```python
from build123d import *
from OCP.BRepFilletAPI import BRepFilletAPI_MakeChamfer

# Parameters (mm, degrees)
SKETCH1_W                 = 41.91
SKETCH1_H                 = 41.91
EXTRUDE1_DEPTH            = 33
SKETCH9_R                 = 11
EXTRUDE5_DEPTH            = 2
SKETCH7_R                 = 2.50063
EXTRUDE3_DEPTH            = 18
F_4_40_TAPPED_HOLE1_D     = 2.2606
F_4_40_TAPPED_HOLE1_DEPTH = 6.41
F_4_40_TAPPED_HOLE1_TIP   = 0.679152758
F_4_40_TAPPED_HOLE2_D     = 2.2606
F_4_40_TAPPED_HOLE2_DEPTH = 29.905
F_4_40_TAPPED_HOLE2_TIP   = 0.679152758
SKETCH14_R                = 3.1
CUT_EXTRUDE1_DEPTH        = 2.6
CHAMFER1_SIZE             = 0.508
CHAMFER2_SIZE             = 4.064
SKETCH16_R                = 3.3147
CUT_EXTRUDE3_DEPTH        = 5.08
BOSS_EXTRUDE1_START       = 4.08
SKETCH17_R                = 2.50063
BOSS_EXTRUDE1_DEPTH       = 4.08
CHAMFER3_SIZE             = 0.254
CHAMFER4_SIZE             = 0.254
CHAMFER4_SIZE2            = 0.205559306
SKETCH18_W                = 5.00126
SKETCH18_H                = 1
CUT_EXTRUDE4_DEPTH        = 15
SKETCH24_R                = 0.5
BOSS_EXTRUDE2_DEPTH       = 19
SKETCH25_R                = 5.83
BOSS_EXTRUDE3_DEPTH       = 14
SKETCH26_R                = 17.29
BOSS_EXTRUDE4_DEPTH       = 11
SKETCH27_R                = 17.29
SKETCH27_R_2              = 5.83
CUT_EXTRUDE5_DEPTH        = 6


with BuildPart() as part:
    # Sketch1 → Extrude1 (new body)
    with BuildSketch(Plane(origin=(0, 0, 0), x_dir=(1, 0, 0), z_dir=(0, 1, 0))):
        Rectangle(SKETCH1_W, SKETCH1_H)
    extrude(amount=-EXTRUDE1_DEPTH)

    # Sketch9 → Extrude5 (add)
    with BuildSketch(Plane(origin=(0, 0, 0), x_dir=(1, 0, 0), z_dir=(0, 1, 0))):
        with Locations(Location((0, 0, 0), (0, 0, 90))):
            Circle(SKETCH9_R)
    extrude(amount=EXTRUDE5_DEPTH)

    # Sketch7 → Extrude3 (add)
    with BuildSketch(Plane(origin=(0, 2, 0), x_dir=(-1, 0, 0), z_dir=(0, 1, 0))):
        with Locations(Location((0, 0, 0), (0, 0, 90))):
            Circle(SKETCH7_R)
    extrude(amount=EXTRUDE3_DEPTH)

    # #4-40 Tapped Hole1
    with Locations(Plane(origin=(0, 0, 0), x_dir=(-1, 0, 0), z_dir=(0, 1, 0))):
        with Locations((15.5, -15.5), (15.5, 15.5), (-15.5, 15.5), (-15.5, -15.5)):
            Hole(F_4_40_TAPPED_HOLE1_D / 2, depth=F_4_40_TAPPED_HOLE1_DEPTH)
            with Locations((0, 0, -(F_4_40_TAPPED_HOLE1_DEPTH + F_4_40_TAPPED_HOLE1_TIP / 2))):  # 118° drill point
                Cone(0, F_4_40_TAPPED_HOLE1_D / 2, F_4_40_TAPPED_HOLE1_TIP, mode=Mode.SUBTRACT)

    # #4-40 Tapped Hole2
    with Locations(Plane.XZ.offset(33)):
        with Locations((15.5, -15.5), (-15.5, 15.5), (-15.5, -15.5), (15.5, 15.5)):
            Hole(F_4_40_TAPPED_HOLE2_D / 2, depth=F_4_40_TAPPED_HOLE2_DEPTH)
            with Locations((0, 0, -(F_4_40_TAPPED_HOLE2_DEPTH + F_4_40_TAPPED_HOLE2_TIP / 2))):  # 118° drill point
                Cone(0, F_4_40_TAPPED_HOLE2_D / 2, F_4_40_TAPPED_HOLE2_TIP, mode=Mode.SUBTRACT)

    # Sketch14 → Cut-Extrude1 (cut)
    with BuildSketch(Plane(origin=(0, -33, 0), x_dir=(1, 0, 0), z_dir=(0, 1, 0))):
        with Locations(Location((15.5, 15.5, 0), (0, 0, 270))):
            Circle(SKETCH14_R)
        with Locations(Location((-15.5, 15.5, 0), (0, 0, 270))):
            Circle(SKETCH14_R)
        with Locations(Location((-15.5, -15.5, 0), (0, 0, 270))):
            Circle(SKETCH14_R)
        with Locations(Location((15.5, -15.5, 0), (0, 0, 270))):
            Circle(SKETCH14_R)
    extrude(amount=CUT_EXTRUDE1_DEPTH, mode=Mode.SUBTRACT)

    # Chamfer1
    chamfer1_edges = [part.edges().sort_by_distance(p)[0] for p in [
        (0, 20, -2.50063),
    ]]
    chamfer(chamfer1_edges, length=CHAMFER1_SIZE)

    # Chamfer2
    chamfer2_edges = [part.edges().sort_by_distance(p)[0] for p in [
        (20.955, -16.5, 20.955),
        (-20.955, -16.5, 20.955),
        (-20.955, -16.5, -20.955),
        (20.955, -16.5, -20.955),
    ]]
    chamfer(chamfer2_edges, length=CHAMFER2_SIZE)

    # Sketch16 → Cut-Extrude3 (cut)
    with BuildSketch(Plane.XZ.offset(33)):
        with Locations(Location((0, 0, 0), (0, 0, 270))):
            Circle(SKETCH16_R)
    extrude(amount=-CUT_EXTRUDE3_DEPTH, mode=Mode.SUBTRACT)

    # Sketch17 → Boss-Extrude1 (add)
    with BuildSketch(Plane.XZ.offset(27.92).offset(BOSS_EXTRUDE1_START)):
        with Locations(Location((0, 0, 0), (0, 0, 90))):
            Circle(SKETCH17_R)
    extrude(amount=-BOSS_EXTRUDE1_DEPTH)

    # Chamfer3
    chamfer3_edges = [part.edges().sort_by_distance(p)[0] for p in [
        (-18.923, -33, 18.923),
        (0, -33, 3.3147),
        (0, -32, -2.50063),
        (-20.955, 0, 0),
        (-20.955, -33, 0),
        (20.955, 0, 0),
        (0, 0, -20.955),
        (0, 0, 20.955),
        (-18.923, 0, -18.923),
        (18.923, 0, -18.923),
        (18.923, 0, 18.923),
        (-18.923, 0, 18.923),
        (0, -33, 20.955),
        (20.955, -33, 0),
        (0, -33, -20.955),
        (-18.923, -33, -18.923),
        (18.923, -33, -18.923),
        (18.923, -33, 18.923),
    ]]
    chamfer(chamfer3_edges, length=CHAMFER3_SIZE)

    # Chamfer4: one chamfer whose edges measure the first distance from different faces: ONE call of the kernel's chamfer builder (chamfer() names one face for all edges)
    chamfer4_edges_1 = [part.edges().sort_by_distance(p)[0] for p in [
        (16.891, -16.5, -20.955),
        (20.955, -16.5, -16.891),
    ]]
    chamfer4_side_1 = [part.faces().sort_by_distance(p)[0] for p in [
        (18.923, -16.5, -18.923),
    ]]
    chamfer4_edges_2 = [part.edges().sort_by_distance(p)[0] for p in [
        (-16.891, -16.5, -20.955),
        (-20.955, -16.5, -16.891),
    ]]
    chamfer4_side_2 = [part.faces().sort_by_distance(p)[0] for p in [
        (-18.923, -16.5, -18.923),
    ]]
    chamfer4_edges_3 = [part.edges().sort_by_distance(p)[0] for p in [
        (20.955, -16.5, 16.891),
        (16.891, -16.5, 20.955),
    ]]
    chamfer4_side_3 = [part.faces().sort_by_distance(p)[0] for p in [
        (18.923, -16.5, 18.923),
    ]]
    chamfer4_edges_4 = [part.edges().sort_by_distance(p)[0] for p in [
        (-16.891, -16.5, 20.955),
        (-20.955, -16.5, 16.891),
    ]]
    chamfer4_side_4 = [part.faces().sort_by_distance(p)[0] for p in [
        (-18.923, -16.5, 18.923),
    ]]
    chamfer4 = BRepFilletAPI_MakeChamfer(part.part.solid().wrapped)
    for e in chamfer4_edges_1:
        chamfer4.Add(CHAMFER4_SIZE, CHAMFER4_SIZE2, e.wrapped, chamfer4_side_1[0].wrapped)  # the first distance lies on this face
    for e in chamfer4_edges_2:
        chamfer4.Add(CHAMFER4_SIZE, CHAMFER4_SIZE2, e.wrapped, chamfer4_side_2[0].wrapped)  # the first distance lies on this face
    for e in chamfer4_edges_3:
        chamfer4.Add(CHAMFER4_SIZE, CHAMFER4_SIZE2, e.wrapped, chamfer4_side_3[0].wrapped)  # the first distance lies on this face
    for e in chamfer4_edges_4:
        chamfer4.Add(CHAMFER4_SIZE, CHAMFER4_SIZE2, e.wrapped, chamfer4_side_4[0].wrapped)  # the first distance lies on this face
    add(Compound.cast(chamfer4.Shape()), mode=Mode.REPLACE)

    # Sketch18 → Cut-Extrude4 (cut)
    with BuildSketch(Plane(origin=(0, 20, 0), x_dir=(1, 0, 0), z_dir=(0, 1, 0))):
        with Locations((0, 2.50063)):
            Rectangle(SKETCH18_W, SKETCH18_H)
    extrude(amount=-CUT_EXTRUDE4_DEPTH, mode=Mode.SUBTRACT)

    # Sketch24 → Boss-Extrude2 (add)
    with BuildSketch(Plane(origin=(20.955, 0, 0), x_dir=(0, 0, -1), z_dir=(1, 0, 0))):
        with Locations((2.4, -30.086520784)):
            Circle(SKETCH24_R)
        with Locations((1.2, -30.086520784)):
            Circle(SKETCH24_R)
        with Locations((0, -30.086520784)):
            Circle(SKETCH24_R)
    extrude(amount=BOSS_EXTRUDE2_DEPTH)

    # Sketch25 → Boss-Extrude3 (add)
    with BuildSketch(Plane(origin=(0, 20, 0), x_dir=(1, 0, 0), z_dir=(0, 1, 0))):
        with Locations(Location((0, 0, 0), (0, 0, 270))):
            Circle(SKETCH25_R)
    extrude(amount=-BOSS_EXTRUDE3_DEPTH)

    # Sketch26 → Boss-Extrude4 (add)
    with BuildSketch(Plane(origin=(0, 20, 0), x_dir=(1, 0, 0), z_dir=(0, 1, 0))):
        with Locations(Location((0, 0, 0), (0, 0, 270))):
            Circle(SKETCH26_R)
    extrude(amount=-BOSS_EXTRUDE4_DEPTH)

    # Sketch27 → Cut-Extrude5 (cut)
    with BuildSketch(Plane(origin=(0, 20, 0), x_dir=(1, 0, 0), z_dir=(0, 1, 0))):
        with Locations(Location((0, 0, 0), (0, 0, 270))):
            Circle(SKETCH27_R)
        with Locations(Location((0, 0, 0), (0, 0, 270))):
            Circle(SKETCH27_R_2, mode=Mode.SUBTRACT)
    extrude(amount=-CUT_EXTRUDE5_DEPTH, mode=Mode.SUBTRACT)


solid = part.part
```
The listing builds one solid part. Answer for the finished solid, in the listing's coordinates (mm). A direction names the side the tool comes from. Round coordinates to 2 decimals unless told otherwise and drop trailing zeros. Loops run counter-clockwise (first coordinate to the right, second up) from the corner with the lowest first, then second, coordinate; pieces in that order, holes last. Notation, with made-up numbers: (12.25, 68) - (33.25, 68) arc R26 ccw to (33.25, 95) - close; hole circle Ø11 at (78, 55). An arc over 180 degrees is marked (long way). Return JSON: item names as keys, results as strings. Group by question number.
1. The part is cut by section D-D on x = 27.5. Determine the outline of the cut face in (y, z).
2. Each of these flat-tipped pins is pushed along its axis until it touches: P1, Ø3.5, axis at x = -15.5, z = 15.5, coming from the +Y side; P2, Ø1.9, axis at x = 16.5, z = 16.5, coming from the -Y side; P3, Ø1.8, axis at x = -15.5, z = -15.5, coming from the -Y side; P4, Ø4, axis at x = 0, z = 0, coming from the -Y side. Where does it stop, or does it pass through?
3. Consider probe 1 along X at (y, z) = (-2, 15.5) (3 decimals); probe 2 along X at (y, z) = (-5, -15) (3 decimals). Determine where each line is inside the solid, lowest interval first.
4. The part is cut by section B-B on x = -15.5. Determine the outline of the cut face in (y, z) (3 decimals), then the cut area to 3 significant figures.
5. The mould has two halves that part along Z. Classify faces 1 (the cylindrical face through (-0.751, -29.86, 2.385)), 2 (the flat face through (-18.86, -0.13, 18.81)), 3 (the flat face through (0, 20, 0)): pulls with the +Z half, pulls with the -Z half, needs draft (parallel to the pull), parting line crosses it, or undercut.
6. The part is cut by section A-A on x = 10. Determine the outline of the cut face in (y, z) (3 decimals), then the cut area to 3 significant figures.
7. Which of the six approach directions +Z, -Z, +X, -X, +Y, -Y give full straight-line access (tool end or side, diameter ignored) to faces 4 (the flat face through (-18.897, -16.273, 18.949)), 5 (the cylindrical face through (10.74, 0.99, 2.38)), 6 (the flat face through (0, -32, 0))?
8. The part is cut by section C-C on y = 10.5. Determine the outline of the cut face in (x, z).
Resolved:
{
 "1": {"outline": "circle Ø1 at (-30.09, -2.4); circle Ø1 at (-30.09, -1.2); circle Ø1 at (-30.09, 0)"},
 "2": {"P1": "stops at y = 0", "P2": "stops at y = -30.4", "P3": "passes through", "P4": "stops at y = -32"},
 "3": {"probe 1": "x = -20.955 to -16.63, -14.37 to 14.37, 16.63 to 20.955", "probe 2": "x = -20.955 to -16.514, -14.486 to 14.486, 16.514 to 20.955"},
 "4": {"outline": "(-33, -20.701) - (-32.746, -20.955) - (-0.254, -20.955) - (0, -20.701) - (0, -16.63) - (-30.4, -16.63) - (-30.4, -18.6) - (-33, -18.6) - close; (-33, -12.4) - (-30.4, -12.4) - (-30.4, -14.37) - (0, -14.37) - (0, 14.37) - (-30.4, 14.37) - (-30.4, 12.4) - (-33, 12.4) - close; (-33, 18.6) - (-30.4, 18.6) - (-30.4, 16.63) - (0, 16.63) - (0, 20.701) - (-0.254, 20.955) - (-32.746, 20.955) - (-33, 20.701) - close; (9, -7.661) - (14, -7.661) - (14, 7.661) - (9, 7.661) - close", "area": "1,290 mm²"},
 "5": {"face 1": "undercut", "face 2": "pulls with the +Z half", "face 3": "needs draft"},
 "6": {"outline": "(-33, -20.701) - (-32.746, -20.955) - (-0.254, -20.955) - (0, -20.701) - (0, -4.583) - (2, -4.583) - (2, 4.583) - (0, 4.583) - (0, 20.701) - (-0.254, 20.955) - (-32.746, 20.955) - (-33, 20.701) - close; (9, -14.105) - (14, -14.105) - (14, 14.105) - (9, 14.105) - close", "area": "1,540 mm²"},
 "7": {"face 4": "+Z, -X, +Y, -Y", "face 5": "none", "face 6": "-Y"},
 "8": {"outline": "circle Ø34.58 at (0, 0)"}
}
